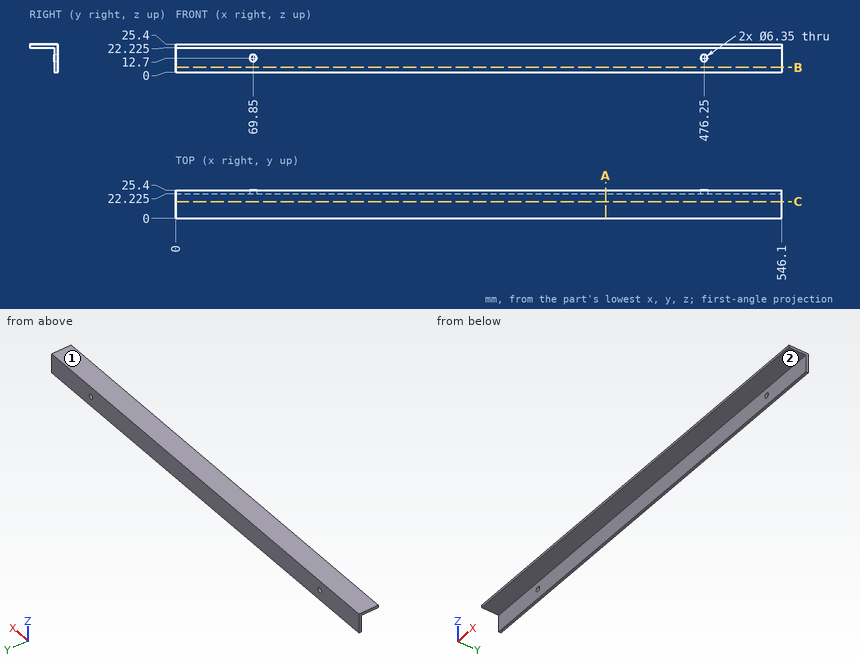
Geometry: see drawing. Coordinates: mm, zero at the bounding-box minimum. A direction names the side the tool comes from. Coordinates: 2 decimals unless noted, no trailing zeros. Loops run counter-clockwise (first coordinate to the right, second up) from the corner with the lowest first, then second, coordinate; pieces in that order, holes last. Notation, with made-up numbers: (5.25, 22.25) - (25.25, 22.25) arc R14 cw to (25.25, 40.25) - close; hole circle Ø4 at (32, 87). An arc over 180 degrees is marked (long way). Answer as CSV lines item,"result".
1. Ray query, line 1 (X direction, y = 23.15, z = 12.7) (3 decimals); line 2 (Z direction, x = 476.25, y = 23.4) (3 decimals); line 3 (Z direction, x = 388, y = 11.75) (3 decimals). Return the intervals inside material, ascending.
Established:
line 1,"x = 0 to 66.675, 73.025 to 473.075, 479.425 to 546.1"
line 2,"z = 0 to 9.525, 15.875 to 25.4"
line 3,"z = 22.225 to 25.4"
2. Contact query for flat-ended pins moving along their axis: pin 1 (6.5 mm diameter, centred on x = 181, y = 13, fed in from -Z) (3 decimals); pin 2 (6 mm diameter, centred on x = 462.5, z = 8, fed in from -Y) (3 decimals). Output: stop coordinate, or through.
Established:
pin 1,"stops at z = 22.225"
pin 2,"stops at y = 22.225"
3. Reachability of the marked faces 1 and 2 from +Z, -Z, +X, -X, +Y, -Y: full face, straight path, thin tool, end or side. Return the list, or none.
Established:
face 1,"+Z, +X, -X, +Y, -Y"
face 2,"-Z, +X, -X, -Y"
4. Section B-B (z = 4.25). Return loops of the section in (x, y) (3 decimals), then the cut area to 3 significant figures.
Established:
outline,"(0, 22.225) - (546.1, 22.225) - (546.1, 25.4) - (0, 25.4) - close"
area,"1,730 mm2"
5. Section A-A (x = 387.5). Return loops of the section in (y, z) (3 decimals), then the cut area to 3 significant figures.
Established:
outline,"(0, 22.225) - (22.225, 22.225) - (22.225, 0) - (25.4, 0) - (25.4, 25.4) - (0, 25.4) - close"
area,"151 mm2"
